Build history of the part. All positions in model axes, mm. A direction names the side the tool comes from. Round coordinates to 2 decimals unless told otherwise and drop trailing zeros. Write each loop counter-clockwise with the first axis right and the second up, starting at its lowest first coordinate (ties: lowest second). Pieces come first, ordered by that corner, then holes.
Item 1: 3-axis set-ups, long thin cutter, end or side, ignore diameter. For faces 4 (the flat face through (200, 9.806, 104)), 5 (the cylindrical face through (-25.07, -4.455, -3.905)), 6 (the flat face through (197, 12.7, 0)), 7 (the flat face through (200, -2, 12.7)), 8 (the flat face through (200, -33, 227.2)): which of +Z, -Z, +X, -X, +Y, -Y reach the whole face in a straight line?
Item 2: Mould opens along X. For faces 1 (the flat face through (200, -11.694, -103)), 2 (the cylindrical face through (228.615, -24.182, 222.27)), 3 (the flat face through (200, -33, -224.2)) say: +X half, -X half, draft (parallel to the pull), parting line (faces both ways), or undercut.
Item 3: Wall check: probe 1 along X at (y, z) = (-9, -91); probe 2 along Z at (x, y) = (198.5, -8); probe 3 along Z at (x, y) = (356, -1.5). Give the ranges that are in metal, low to high.
Item 4: Drop flat-ended pins along their axis: pin 1 Ø5 at (x, z) = (215.5, -49) entering from +Y; pin 2 Ø3 at (y, z) = (421, -42.5) entering from +X; pin 3 Ø18.5 at (x, z) = (194.5, -73.5) entering from -Y; pin 4 Ø5 at (x, z) = (346, -285) entering from -Y. Give the stop position or say it passes through.
Item 5: Band-saw the part on B-B, the plane z = -270. Write the cut outline in (x, y), then the cut area to 3 significant figures.
Item 6: Band-saw the part on A-A, the plane x = 251.5. Write the cut outline in (y, z).
Item 7: Band-saw the part on C-C, the plane y = 80.5. Write the cut outline in (x, z), then the cut area to 3 significant figures.
```python
from build123d import *

# Parameters (mm, degrees)
SKETCH1_W                = 28.4
SKETCH1_H                = 28.4
SKETCH1_W_2              = 25.4
SKETCH1_H_2              = 25.4
EXTRUDE_THIN1_DEPTH      = 400
SKETCH2_W                = 23
SKETCH2_H                = 23
SKETCH2_W_2              = 20
SKETCH2_H_2              = 20
EXTRUDE_THIN2_DEPTH      = 183
EXTRUDE_THIN2_DEPTH_BACK = 208.4
SKETCH3_W                = 60
SKETCH3_H                = 28.4
BOSS_EXTRUDE1_DEPTH      = 30
SKETCH4_W                = 23
SKETCH4_H                = 60
BOSS_EXTRUDE2_DEPTH      = 30
SKETCH5_R                = 5
BOSS_EXTRUDE3_DEPTH      = 30
SKETCH6_R                = 5
BOSS_EXTRUDE4_DEPTH      = 30
SKETCH7_R                = 5
BOSS_EXTRUDE5_DEPTH      = 30
SKETCH8_R                = 5
BOSS_EXTRUDE6_DEPTH      = 30
BOSS_EXTRUDE7_DEPTH      = 400
SKETCH10_W               = 372.349277715
SKETCH10_H               = 4
BOSS_EXTRUDE8_DEPTH      = 5
SKETCH11_W               = 380
SKETCH11_H               = 8
BOSS_EXTRUDE9_DEPTH      = 5
SKETCH12_W               = 27.915252313
SKETCH12_H               = 18.485240527
BOSS_EXTRUDE10_DEPTH     = 40
SKETCH13_R               = 3
BOSS_EXTRUDE11_DEPTH     = 60
SKETCH14_W               = 4.655382852
SKETCH14_H               = 68.075309474
SKETCH14_W_2             = 4.976973146
BOSS_EXTRUDE12_DEPTH     = 2.5
SKETCH15_W               = 37.547608311
SKETCH15_H               = 6.653489581
BOSS_EXTRUDE13_DEPTH     = 30
SKETCH16_W               = 11.532338845
SKETCH16_H               = 6.653489581
BOSS_EXTRUDE14_DEPTH     = 16
SKETCH17_W               = 10.054157613
SKETCH17_H               = 12.862513988
BOSS_EXTRUDE15_DEPTH     = 30
SKETCH18_R               = 3
BOSS_EXTRUDE16_DEPTH     = 120
SKETCH19_W               = 380
SKETCH19_H               = 8
BOSS_EXTRUDE17_DEPTH     = 5
SKETCH22_W               = 15
SKETCH22_H               = 5
BOSS_EXTRUDE18_DEPTH     = 350
SKETCH23_W               = 21.129059452
SKETCH23_H               = 9.044463221
SKETCH23_W_2             = 31.579735641
BOSS_EXTRUDE19_DEPTH     = 10
SKETCH24_R               = 30
BOSS_EXTRUDE20_DEPTH     = 10
SKETCH25_R               = 30
BOSS_EXTRUDE21_DEPTH     = 10
SKETCH26_R               = 30
BOSS_EXTRUDE22_DEPTH     = 10
SKETCH27_R               = 30
BOSS_EXTRUDE23_DEPTH     = 10


with BuildPart() as part:
    # Sketch1 → Extrude-Thin1 (new body)
    with BuildSketch(Plane(origin=(0, 0, 0), x_dir=(0, 0, -1), z_dir=(1, 0, 0))):
        Rectangle(SKETCH1_W, SKETCH1_H)
        Rectangle(SKETCH1_W_2, SKETCH1_H_2, mode=Mode.SUBTRACT)
    extrude(amount=EXTRUDE_THIN1_DEPTH)

    # Sketch2 → Extrude-Thin2 (add, two sides)
    with BuildSketch(Plane.XY.offset(14.2)) as extrude_thin2_sk:
        with Locations((200, -1.693644648)):
            Rectangle(SKETCH2_W, SKETCH2_H)
        with Locations((200, -1.693644648)):
            Rectangle(SKETCH2_W_2, SKETCH2_H_2, mode=Mode.SUBTRACT)
    extrude(amount=EXTRUDE_THIN2_DEPTH)
    extrude(extrude_thin2_sk.sketch, amount=-EXTRUDE_THIN2_DEPTH_BACK)

    # Sketch3 → Boss-Extrude1 (add)
    with BuildSketch(Plane(origin=(0, -14.2, 0), x_dir=(-1, 0, 0), z_dir=(0, -1, 0))):
        with Locations((-370, 0)):
            Rectangle(SKETCH3_W, SKETCH3_H)
        with Locations((-30, 0)):
            Rectangle(SKETCH3_W, SKETCH3_H)
    extrude(amount=BOSS_EXTRUDE1_DEPTH)

    # Sketch4 → Boss-Extrude2 (add)
    with BuildSketch(Plane(origin=(0, -13.193644648, 0), x_dir=(-1, 0, 0), z_dir=(0, -1, 0))):
        with Locations((-200, -167.2)):
            Rectangle(SKETCH4_W, SKETCH4_H)
        with Locations((-200, 164.2)):
            Rectangle(SKETCH4_W, SKETCH4_H)
    extrude(amount=BOSS_EXTRUDE2_DEPTH)

    # Sketch5 → Boss-Extrude3 (add)
    with BuildSketch(Plane(origin=(400, 0, 0), x_dir=(0, 0, -1), z_dir=(1, 0, 0))):
        with Locations((0, -34.2)):
            Circle(SKETCH5_R)
    extrude(amount=BOSS_EXTRUDE3_DEPTH)

    # Sketch6 → Boss-Extrude4 (add)
    with BuildSketch(Plane(origin=(0, 0, -194.2), x_dir=(-1, 0, 0), z_dir=(0, 0, -1))):
        with Locations((-200, -33.193644648)):
            Circle(SKETCH6_R)
    extrude(amount=BOSS_EXTRUDE4_DEPTH)

    # Sketch7 → Boss-Extrude5 (add)
    with BuildSketch(Plane.ZY):
        with Locations((0, -34.2)):
            Circle(SKETCH7_R)
    extrude(amount=BOSS_EXTRUDE5_DEPTH)

    # Sketch8 → Boss-Extrude6 (add)
    with BuildSketch(Plane.XY.offset(197.2)):
        with Locations((200, -33.193644648)):
            Circle(SKETCH8_R)
    extrude(amount=BOSS_EXTRUDE6_DEPTH)

    # Sketch9 → Boss-Extrude7 (add)
    with BuildSketch(Plane(origin=(0, 14.2, 0), x_dir=(1, 0, 0), z_dir=(0, 1, 0))):
        Polygon((10, 3.8), (20, 3.8), (20, 1.8), (13.177515759, 1.8), (13.177515759, -2.2), (20, -2.2), (20, -4.2), (10, -4.2), align=None)
        Polygon((380, 3.8), (390, 3.8), (390, -4.2), (380, -4.2), (380, -2.2), (385.526793474, -2.2), (385.526793474, 1.8), (380, 1.8), align=None)
    extrude(amount=BOSS_EXTRUDE7_DEPTH)

    # Sketch10 → Boss-Extrude8 (add)
    with BuildSketch(Plane(origin=(0, 264.2, 0), x_dir=(1, 0, 0), z_dir=(0, 1, 0))):
        with Locations((199.352154617, -0.2)):
            Rectangle(SKETCH10_W, SKETCH10_H)
    extrude(amount=BOSS_EXTRUDE8_DEPTH)

    # Sketch11 → Boss-Extrude9 (add)
    with BuildSketch(Plane(origin=(0, 414.2, 0), x_dir=(1, 0, 0), z_dir=(0, 1, 0))):
        with Locations((200, -0.2)):
            Rectangle(SKETCH11_W, SKETCH11_H)
    extrude(amount=BOSS_EXTRUDE9_DEPTH)

    # Sketch12 → Boss-Extrude10 (add)
    with BuildSketch(Plane.XY.offset(4.2)):
        with Locations((199.518702547, 409.957379737)):
            Rectangle(SKETCH12_W, SKETCH12_H)
    extrude(amount=BOSS_EXTRUDE10_DEPTH)

    # Sketch13 → Boss-Extrude11 (add)
    with BuildSketch(Plane(origin=(0, 0, 4.2), x_dir=(-1, 0, 0), z_dir=(0, 0, -1))):
        with Locations((-198.49073191, 410.167255752)):
            Circle(SKETCH13_R)
    extrude(amount=BOSS_EXTRUDE11_DEPTH)

    # Sketch14 → Boss-Extrude12 (add)
    with BuildSketch(Plane(origin=(0, 419.2, 0), x_dir=(1, 0, 0), z_dir=(0, 1, 0))):
        with Locations((215.804020129, 29.837654737)):
            Rectangle(SKETCH14_W, SKETCH14_H)
        with Locations((183.072589817, 29.837654737)):
            Rectangle(SKETCH14_W_2, SKETCH14_H)
    extrude(amount=BOSS_EXTRUDE12_DEPTH)

    # Sketch15 → Boss-Extrude13 (add)
    with BuildSketch(Plane(origin=(0, 421.7, 0), x_dir=(1, 0, 0), z_dir=(0, 1, 0))):
        with Locations((199.357907399, 26.510909946)):
            Rectangle(SKETCH15_W, SKETCH15_H)
    extrude(amount=BOSS_EXTRUDE13_DEPTH)

    # Sketch16 → Boss-Extrude14 (add)
    with BuildSketch(Plane(origin=(0, 421.7, 0), x_dir=(-1, 0, 0), z_dir=(0, -1, 0))):
        with Locations((-198.059420633, 26.510909946)):
            Rectangle(SKETCH16_W, SKETCH16_H)
    extrude(amount=BOSS_EXTRUDE14_DEPTH)

    # Sketch17 → Boss-Extrude15 (add)
    with BuildSketch(Plane(origin=(0, 264.2, 0), x_dir=(-1, 0, 0), z_dir=(0, -1, 0))):
        with Locations((-200.355829852, 0)):
            Rectangle(SKETCH17_W, SKETCH17_H)
    extrude(amount=BOSS_EXTRUDE15_DEPTH)

    # Sketch18 → Boss-Extrude16 (add)
    with BuildSketch(Plane(origin=(0, 264.2, 0), x_dir=(1, 0, 0), z_dir=(0, 1, 0))):
        with Locations((198.604681124, 0)):
            Circle(SKETCH18_R)
    extrude(amount=BOSS_EXTRUDE16_DEPTH)

    # Sketch19 → Boss-Extrude17 (add)
    with BuildSketch(Plane(origin=(0, 349.2, 0), x_dir=(1, 0, 0), z_dir=(0, 1, 0))):
        with Locations((200, -0.2)):
            Rectangle(SKETCH19_W, SKETCH19_H)
    extrude(amount=BOSS_EXTRUDE17_DEPTH)

    # Sketch22 → Boss-Extrude18 (add)
    with BuildSketch(Plane(origin=(0, 0, -3.8), x_dir=(-1, 0, 0), z_dir=(0, 0, -1))):
        with Locations((-357.561728319, 351.7)):
            Rectangle(SKETCH22_W, SKETCH22_H)
        with Locations((-57.561728319, 351.7)):
            Rectangle(SKETCH22_W, SKETCH22_H)
    extrude(amount=BOSS_EXTRUDE18_DEPTH)

    # Sketch23 → Boss-Extrude19 (add)
    with BuildSketch(Plane(origin=(0, 0, -353.8), x_dir=(-1, 0, 0), z_dir=(0, 0, -1))):
        with Locations((-58.848339235, 350.994945207)):
            Rectangle(SKETCH23_W, SKETCH23_H)
        with Locations((-357.551157011, 350.994945207)):
            Rectangle(SKETCH23_W_2, SKETCH23_H)
    extrude(amount=BOSS_EXTRUDE19_DEPTH)

    # Sketch24 → Boss-Extrude20 (add)
    with BuildSketch(Plane(origin=(0, 0, -224.2), x_dir=(-1, 0, 0), z_dir=(0, 0, -1))):
        with Locations((-200, -33.193644648)):
            Circle(SKETCH24_R)
    extrude(amount=-BOSS_EXTRUDE20_DEPTH)

    # Sketch25 → Boss-Extrude21 (add)
    with BuildSketch(Plane.ZY.offset(30)):
        with Locations((0, -34.2)):
            Circle(SKETCH25_R)
    extrude(amount=-BOSS_EXTRUDE21_DEPTH)

    # Sketch26 → Boss-Extrude22 (add)
    with BuildSketch(Plane.XY.offset(227.2)):
        with Locations((200, -33.193644648)):
            Circle(SKETCH26_R)
    extrude(amount=-BOSS_EXTRUDE22_DEPTH)

    # Sketch27 → Boss-Extrude23 (add)
    with BuildSketch(Plane(origin=(430, 0, 0), x_dir=(0, 0, -1), z_dir=(1, 0, 0))):
        with Locations((0, -34.2)):
            Circle(SKETCH27_R)
    extrude(amount=-BOSS_EXTRUDE23_DEPTH)


solid = part.part
```
Results:
1. face 4: +Z, +X, -X
1. face 5: -X
1. face 6: +X, -X
1. face 7: none
1. face 8: +Z, +X, -X, +Y, -Y
2. face 1: undercut
2. face 2: parting line
2. face 3: draft
3. probe 1: x = 188.5 to 190, 210 to 211.5
3. probe 2: z = -224.2 to -214.2, -14.2 to -12.7, 12.7 to 14.2, 217.2 to 227.2
3. probe 3: z = -14.2 to -12.7, 12.7 to 14.2
4. pin 1: stops at y = 421.7
4. pin 2: stops at x = 218.13
4. pin 3: stops at y = -13.19
4. pin 4: passes through
5. outline: (50.06, 349.2) - (65.06, 349.2) - (65.06, 354.2) - (50.06, 354.2) - close; (350.06, 349.2) - (365.06, 349.2) - (365.06, 354.2) - (350.06, 354.2) - close
5. area: 150 mm2
6. outline: (-14.2, -14.2) - (14.2, -14.2) - (14.2, 14.2) - (-14.2, 14.2) - close; (264.2, -1.8) - (269.2, -1.8) - (269.2, 2.2) - (264.2, 2.2) - close; (349.2, -3.8) - (354.2, -3.8) - (354.2, 4.2) - (349.2, 4.2) - close; (414.2, -3.8) - (419.2, -3.8) - (419.2, 4.2) - (414.2, 4.2) - close; hole (-12.7, -12.7) - (12.7, -12.7) - (12.7, 12.7) - (-12.7, 12.7) - close
7. outline: (10, -3.8) - (20, -3.8) - (20, -1.8) - (13.18, -1.8) - (13.18, 2.2) - (20, 2.2) - (20, 4.2) - (10, 4.2) - close; (380, -3.8) - (390, -3.8) - (390, 4.2) - (380, 4.2) - (380, 2.2) - (385.53, 2.2) - (385.53, -1.8) - (380, -1.8) - close
7. area: 111 mm2
